Input: part model. Units: mm. Frame: model coordinates. Face numbers are marked on the shaded views. A direction names the side the tool comes from. Coordinates: 2 decimals unless noted, no trailing zeros. Write each loop counter-clockwise with the first axis right and the second up, starting at its lowest first coordinate (ties: lowest second). Pieces come first, ordered by that corner, then holes. Notation, with made-up numbers: (66, 83.5) -> (96, 83.5) arc R31 ccw to (96, 109.5) -> close; hole circle Ø8 at (8.5, -38.75). An arc over 180 degrees is marked (long way). Use one line per item in the form item = value. Start each with the question number.
(1) Pull-direction query (X, two-part tool) for the marked faces 1, 2 and 3; classes: released by +X, released by -X, zero draft, split by the parting line, or undercut.
(2) Ray query, line 1 along X through (y, z) = (0, 3); line 2 along X through (y, z) = (0, -4.45); line 3 along Y through (x, z) = (-9.55, 4.5). Return the intervals inside material, ascending.
(3) Set-up query: the marked faces 4 and 5. Return all of +Z, -Z, +X, -X, +Y, -Y with unobstructed straight access to the full face (end or side cutting, diameter ignored); none if empty.
(4) First-contact query: pin 1 (12 mm diameter, centred on x = 2, y = -0.5, fed in from -Z); pin 2 (2 mm diameter, centred on x = -23.5, z = 2, fed in from +Y); pin 3 (10 mm diameter, centred on x = -15.5, z = 7.5, fed in from +Y). Flat tips, straight axial feed; report the tip coordinate or a pass-through.
(5) Cut plane D-D on z = -4.75. Return the cut outline in (x, y), plus the area to 3 significant figures.
(6) Cut plane A-A on y = 0. Return the cut outline in (x, z).
(7) Cut plane C-C on x = 0. Return the cut outline in (y, z).
(8) Cut plane B-B on z = 4. Return the cut outline in (x, y), plus the area to 3 significant figures.
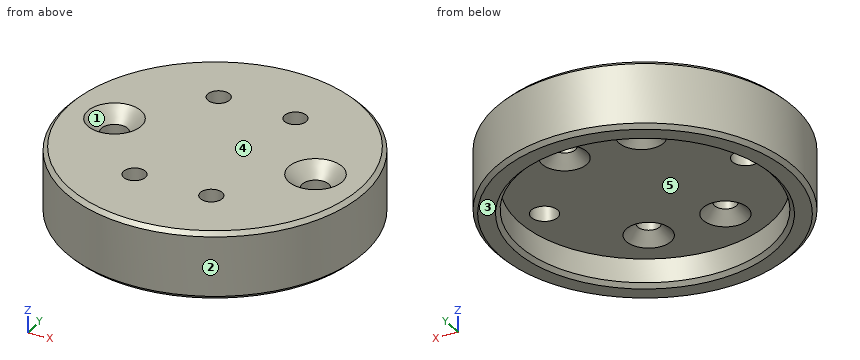
```python
from build123d import *

# Parameters (mm, degrees)
F2_SIZE        = 1
F4_D           = 6.6
F4_CSINK_D     = 13.44
F4_CSINK_ANGLE = 90
F6_D           = 5.5
F6_CSINK_D     = 11.2
F6_CSINK_ANGLE = 90


with BuildPart() as f1:
    # F0 (on Front) → F1 (revolve)
    with BuildSketch(Plane.XZ):
        Polygon((0, 10), (0, 0), (31.6, 0), (31.6, -7), (37.5, -7), (37.5, 10), align=None)
    revolve(axis=Axis((0, 0, 5), (0, 0, -1)))

    # F2
    f2_edges = [f1.edges().sort_by_distance(p)[0] for p in [
        (-31.6, 0, -7),
        (-37.5, 0, -7),
        (-37.5, 0, 10),
    ]]
    chamfer(f2_edges, length=F2_SIZE)

    # F4 (through all)
    with Locations(Plane.XY.offset(10)):
        with Locations((-25, 0), (25, 0)):
            CounterSinkHole(F4_D / 2, F4_CSINK_D / 2, counter_sink_angle=F4_CSINK_ANGLE)

    # F6 (through all)
    with Locations(Plane(origin=(0, 0, 0), x_dir=(1, 0, 0), z_dir=(0, 0, -1))):
        with Locations((-9.55, 19.05), (9.55, 19.05), (9.55, -19.05), (-9.55, -19.05)):
            CounterSinkHole(F6_D / 2, F6_CSINK_D / 2, counter_sink_angle=F6_CSINK_ANGLE)


solid = f1.part
```
Values:
q1.face_1 = undercut
q1.face_2 = split by the parting line
q1.face_3 = zero draft
q2.line_1 = -37.5 to -28.3, -21.7 to 21.7, 28.3 to 37.5
q2.line_2 = -37.5 to -31.6, 31.6 to 37.5
q2.line_3 = -36.26 to -21.8, -16.3 to 16.3, 21.8 to 36.26
q3.face_4 = +Z, +X, -X, +Y, -Y
q3.face_5 = -Z
q4.pin_1 = 0
q4.pin_2 = 30
q4.pin_3 = 36
q5.outline = circle Ø75 at (0, 0); hole circle Ø63.2 at (0, 0)
q5.area = 1,280 mm2
q6.outline = (-37.5, -6) -> (-36.5, -7) -> (-32.6, -7) -> (-31.6, -6) -> (-31.6, 0) -> (-28.3, 0) -> (-28.3, 6.58) -> (-31.72, 10) -> (-36.5, 10) -> (-37.5, 9) -> close; (-21.7, 0) -> (21.7, 0) -> (21.7, 6.58) -> (18.28, 10) -> (-18.28, 10) -> (-21.7, 6.58) -> close; (28.3, 0) -> (31.6, 0) -> (31.6, -6) -> (32.6, -7) -> (36.5, -7) -> (37.5, -6) -> (37.5, 9) -> (36.5, 10) -> (31.72, 10) -> (28.3, 6.58) -> close
q7.outline = (-37.5, -6) -> (-36.5, -7) -> (-32.6, -7) -> (-31.6, -6) -> (-31.6, 0) -> (31.6, 0) -> (31.6, -6) -> (32.6, -7) -> (36.5, -7) -> (37.5, -6) -> (37.5, 9) -> (36.5, 10) -> (-36.5, 10) -> (-37.5, 9) -> close
q8.outline = circle Ø75 at (0, 0); hole circle Ø6.6 at (-25, 0); hole circle Ø5.5 at (-9.55, -19.05); hole circle Ø5.5 at (-9.55, 19.05); hole circle Ø5.5 at (9.55, -19.05); hole circle Ø5.5 at (9.55, 19.05); hole circle Ø6.6 at (25, 0)
q8.area = 4,250 mm2
